Autodesk Inventor part; units mm, degrees
ref_plane "YZ Plane" through (0, 0, 0) normal (1, 0, 0) x (0, 1, 0)
ref_plane "XZ Plane" through (0, 0, 0) normal (0, 1, 0) x (-1, 0, 0)
ref_plane "XY Plane" through (0, 0, 0) normal (0, 0, 1) x (1, 0, 0)
sketch "Sketch1" plane through (0, 0, 0) normal (0, 0, 1) x (1, 0, 0)
  line L0 (-490, 48) -> (490, 48)
  line L1 (490, 48) -> (490, 0)
  line L2 (490, 0) -> (-490, 0)
  line L3 (-490, 0) -> (-490, 48)
  point P0 (0, 0)
  point P1 (0, 0)
  dimension "d0" = 980
  dimension "d1" = 48
extrude "Plate1" add sketch "Sketch1" along normal blind 2
sketch "Sketch2" plane through (490, -2, 0) normal (0, 1, 0) x (-1, 0, 0)
  line L0 (980, 0) -> (0, 0)
  line L1 (0, 0) -> (0, 20)
  line L2 (0, 20) -> (980, 20)
  line L3 (980, 20) -> (980, 0)
edge flange "Flange1" height 20 angle 90 thickness 2 bend radius 2.75 thickness toward (0, 1, 0) relief round relief width 2 relief depth 1 edges at (0, 0, 2) wall of the first edge with corners at (-490, -2, 0) (490, -2, 0) (490, -2, 20) (-490, -2, 20)
bend "Bend1"
corner "Corner1"
sketch "Sketch5" plane through (0, 0, 0) normal (0, 0, -1) x (-1, 0, 0)
  line L0 (490, 48) -> (-490, 48)
  line L1 (490, -2) -> (-490, -2)
  circle A0 centre (0, 48) radius 17.5
  line L2 (243.95, 48) -> (246.05, 48)
  line L3 (246.05, 48) -> (246.05, 26)
  line L4 (246.05, 26) -> (243.95, 26)
  line L5 (243.95, 26) -> (243.95, 48)
  line L6 (-243.95, 48) -> (-246.05, 48)
  line L7 (-246.05, 48) -> (-246.05, 26)
  line L8 (-246.05, 26) -> (-243.95, 26)
  line L9 (-243.95, 26) -> (-243.95, 48)
  line L10 (0, 48) -> (0, -2) construction
  line L11 (490, -2) -> (490, 48)
  line L12 (-490, -2) -> (-490, 48)
  circle A1 centre (-490, 48) radius 17.5
  circle A2 centre (490, 48) radius 17.5
  point P0 (0, 0)
  point P1 (245, 26)
  point P2 (-245, 26)
  point P3 (246.05, 48)
  point P4 (-17.5, 48)
  point P5 (17.5, 48)
  point P6 (-246.05, 48)
  point P7 (472.5, 48)
  point P8 (490, 30.5)
  point P9 (-490, 30.5)
  point P10 (-472.5, 48)
  dimension "d45" = 35
  dimension "d48" = 2.1
  dimension "d49" = 490
  dimension "d51" = 28
  dimension "d52" = 22
extrude "Extrusion1" cut sketch "Sketch5" against normal through all contours L3 L4 L5 L0 | L0 L11 A2 | L9 L8 L7 L0 | L12 L0 A1 picked at (488.702, 36.4796) picked at (-478.4796, 46.702)
sketch "Sketch9" plane through (0, 0, 2) normal (0, 0, 1) x (1, 0, 0)
  line L0 (448.2795, 24.3045) -> (448.2795, 12.3045) construction
  line L1 (448.2795, 12.3045) -> (248.2795, 12.3045) construction
  line L2 (248.2795, 12.3045) -> (248.2795, 24.3045) construction
  line L3 (248.2795, 24.3045) -> (448.2795, 24.3045) construction
  line L4 (-490, 48) -> (490, 48)
  point P0 (0, 0)
  point P1 (1.05, 68)
  point P2 (490, 48)
  point P3 (-490, 48)
  dimension "d40" = 200
  dimension "d41" = 12
mark "Mark2"
equation "\"d2\" = Thickness"
equation "\"d3\" = BendReliefWidth"
equation "\"d4\" = BendReliefDepth"
equation "\"d5\" = MinimumRemnant"
equation "\"d6\" = TransitionRadius"
equation "\"d9\" = BendRadius"
equation "\"d10\" = CornerReliefSize"
equation "\"d11\" = GapSize"
equation "\"d12\" = JacobiRadiusSize"
equation "\"BendReliefWidth\" = Thickness"
equation "\"BendReliefDepth\" = 0.5 * Thickness"
equation "\"CornerReliefSize\" = 4 * Thickness"
equation "\"MinimumRemnant\" = 2 * Thickness"
equation "\"TransitionRadius\" = BendRadius"
equation "\"JacobiRadiusSize\" = BendRadius"
equation "\"GapSize\" = Thickness"
properties part number "MSC 326 STRINGER BOARD  ##" material "Stainless Steel"
Design review of the part built by this model. Coordinates are the model's own, in mm. A direction names the side the tool comes from. Coordinates: 2 decimals unless noted, no trailing zeros. Order: outer loops, then holes, each group sorted by start corner. A loop starts at its lowest first (then second) coordinate and runs counter-clockwise, first axis right, second up. Notation, with made-up numbers: M 16,8.25 L 57,8.25 A14 cw 57,13.25 Z; hole C 85.25,-20 d1. An arc over 180 degrees is marked long. Answer as a JSON object with one key per item and string values. Group by question number.
1) Add section C-C, the plane z = 9.75. Write out the cut boundary in (x, y).
2) For pin 1 (13.5 mm diameter, centred on x = -150.5, y = 23, fed in from +Z); pin 2 (0.6 mm diameter, centred on y = 42, z = 1.5, fed in from -X); pin 3 (1.6 mm diameter, centred on y = 39, z = 1, fed in from +X), all flat-tipped, find the tip position at first contact; note any pin that passes through.
3) Wall thickness on L1, parallel to Y at x = -367.5, z = 13.5; L2, parallel to Z at x = -137, y = 29; L3, parallel to Y at x = -112.5, z = 3.75: over which ranges is each line inside the solid? List them lowest first.
4) Add section A-A, the plane x = 308.5. Write out the cut boundary in (y, z).
5) Add section B-B, the plane y = 11. Write out the cut boundary in (x, z).
6) Tool access review of faces 1 (the flat face through (7, -2, 12)), 2 (the flat face through (7, 0, 12)): name each direction out of +Z, -Z, +X, -X, +Y, -Y from which nothing blocks a thin tool from reaching the whole face with its end or side.
Computed values:
{
 "1": {"outline": "M -490,-2 L 490,-2 L 490,0 L -490,0 Z"},
 "2": {"pin 1": "stops at z = 2", "pin 2": "stops at x = -473.67", "pin 3": "stops at x = 475.5"},
 "3": {"L1": "y = -2 to 0", "L2": "z = 0 to 2", "L3": "y = -1.89 to 0.19"},
 "4": {"outline": "M -2,4.75 A4.75 ccw 2.75,0 L 48,0 L 48,2 L 2.75,2 A2.75 cw 0,4.75 L 0,20 L -2,20 Z"},
 "5": {"outline": "M -490,0 L 490,0 L 490,2 L -490,2 Z"},
 "6": {"face 1": "+Z, -Z, +X, -X, -Y", "face 2": "+Z, +X, -X, +Y"}
}
